from build123d import *

# Parameters (mm, degrees)
SKETCH1_W           = 28
SKETCH1_H           = 28
BOSS_EXTRUDE1_DEPTH = 25
SKETCH2_W           = 28
SKETCH2_H           = 22
CUT_EXTRUDE1_DEPTH  = 22
SKETCH3_W           = 6.8
SKETCH3_H           = 22
CUT_EXTRUDE2_DEPTH  = 46.299006612
SKETCH4_R           = 2.4
CUT_EXTRUDE3_DEPTH  = 44.508619836
SKETCH5_W           = 28
SKETCH5_H           = 6
CUT_EXTRUDE4_DEPTH  = 4
SKETCH6_W           = 2
SKETCH6_H           = 21
CUT_EXTRUDE5_DEPTH  = 45.821869662
SKETCH7_W           = 28
SKETCH7_H           = 26
BOSS_EXTRUDE2_DEPTH = 12
SKETCH9_W           = 6.8
SKETCH9_H           = 22
CUT_EXTRUDE6_DEPTH  = 12
SKETCH10_W          = 28
SKETCH10_H          = 22
CUT_EXTRUDE7_DEPTH  = 12


with BuildPart() as part:
    # Sketch1 → Boss-Extrude1 (new body)
    with BuildSketch(Plane(origin=(0, 0, 0), x_dir=(1, 0, 0), z_dir=(0, 1, 0))):
        with Locations((14, -14)):
            Rectangle(SKETCH1_W, SKETCH1_H)
    extrude(amount=BOSS_EXTRUDE1_DEPTH)

    # Sketch2 → Cut-Extrude1 (cut)
    with BuildSketch(Plane(origin=(0, 25, 0), x_dir=(1, 0, 0), z_dir=(0, 1, 0))):
        with Locations((14, -11)):
            Rectangle(SKETCH2_W, SKETCH2_H)
    extrude(amount=-CUT_EXTRUDE1_DEPTH, mode=Mode.SUBTRACT)

    # Sketch3 → Cut-Extrude2 (cut, through all)
    with BuildSketch(Plane(origin=(0, 3, 0), x_dir=(1, 0, 0), z_dir=(0, 1, 0))):
        with Locations((14, -11)):
            Rectangle(SKETCH3_W, SKETCH3_H)
    extrude(amount=-CUT_EXTRUDE2_DEPTH, mode=Mode.SUBTRACT)

    # Sketch4 → Cut-Extrude3 (cut, through all)
    with BuildSketch(Plane(origin=(0, 0, 22), x_dir=(-1, 0, 0), z_dir=(0, 0, -1))):
        with Locations((-14, 10)):
            Circle(SKETCH4_R)
    extrude(amount=-CUT_EXTRUDE3_DEPTH, mode=Mode.SUBTRACT)

    # Sketch5 → Cut-Extrude4 (cut)
    with BuildSketch(Plane(origin=(0, 25, 0), x_dir=(1, 0, 0), z_dir=(0, 1, 0))):
        with Locations((14, -25)):
            Rectangle(SKETCH5_W, SKETCH5_H)
    extrude(amount=-CUT_EXTRUDE4_DEPTH, mode=Mode.SUBTRACT)

    # Sketch6 → Cut-Extrude5 (cut, through all)
    with BuildSketch(Plane(origin=(28, 0, 0), x_dir=(0, 0, -1), z_dir=(1, 0, 0))):
        with Locations((-27, 10.5)):
            Rectangle(SKETCH6_W, SKETCH6_H)
    extrude(amount=-CUT_EXTRUDE5_DEPTH, mode=Mode.SUBTRACT)

    # Sketch7 → Boss-Extrude2 (add)
    with BuildSketch(Plane.XZ):
        with Locations((14, 13)):
            Rectangle(SKETCH7_W, SKETCH7_H)
    extrude(amount=BOSS_EXTRUDE2_DEPTH)

    # Sketch9 → Cut-Extrude6 (cut)
    with BuildSketch(Plane(origin=(0, 0, 0), x_dir=(1, 0, 0), z_dir=(0, 1, 0))):
        with Locations((14, -11)):
            Rectangle(SKETCH9_W, SKETCH9_H)
    extrude(amount=-CUT_EXTRUDE6_DEPTH, mode=Mode.SUBTRACT)

    # Sketch10 → Cut-Extrude7 (cut)
    with BuildSketch(Plane(origin=(0, 3, 0), x_dir=(1, 0, 0), z_dir=(0, 1, 0))):
        with Locations((14, -11)):
            Rectangle(SKETCH10_W, SKETCH10_H)
    extrude(amount=-CUT_EXTRUDE7_DEPTH, mode=Mode.SUBTRACT)


solid = part.part
Could you check a few things on this model? Use its own coordinates, in mm. A direction names the side the tool comes from. Round coordinates to 2 decimals unless told otherwise and drop trailing zeros. Order: outer loops, then holes, each group sorted by start corner. A loop starts at its lowest first (then second) coordinate and runs counter-clockwise, first axis right, second up.
Q1. Imagine slicing it at D-D, the plane y = 2. List the corners of the cut face in (x, z) for me.
Geometry says:
outline: (0, 22) - (28, 22) - (28, 26) - (0, 26) - close
Q2. Thinking about a two-plate mould opening in Y: for faces 1 (the face through (16.398, 10.106, 23.972)), 2 (the face through (14, 5, 22)), 3 (the face through (14, 21, 24)), which applies, released by +Y, released by -Y, zero draft, split by the parting line, or undercut?
Geometry says:
face 1: undercut
face 2: zero draft
face 3: released by +Y
Q3. Imagine slicing it at C-C, the plane x = 23.75. List the corners of the cut face in (y, z) for me.
Geometry says:
outline: (-12, 0) - (-9, 0) - (-9, 22) - (21, 22) - (21, 26) - (-12, 26) - close
Q4. I'm going to push flat-ended pins straight in: P1, Ø8, axis at x = 10, y = 11, coming from the -Z side; P2, Ø8.5, axis at x = 3, z = 6.5, coming from the +Y side; P3, Ø12, axis at y = 1, z = 7, coming from the +X side; P4, Ø7.5, axis at x = 14, y = 10, coming from the +Z side. Where does each tip first touch, or does it pass through?
Geometry says:
P1: stops at z = 22
P2: stops at y = -9
P3: passes through
P4: stops at z = 26
Q5. Which directions (+Z, -Z, +X, -X, +Y, -Y) give clear straight access to the entire face, cutting with the end or side of a thin tool? Please do faces 4 (the face through (8, -12, 13)), 5 (the face through (10.6, -10, 11)), 6 (the face through (23, -9, 11)).
Geometry says:
face 4: +Z, -Z, +X, -X, -Y
face 5: -Z, +Y, -Y
face 6: -Z, +X, -X, +Y
Q6. Imagine slicing it at A-A, the plane y = 10. List the corners of the cut face in (x, z) for me.
Geometry says:
outline: (0, 22) - (11.6, 22) - (11.6, 26) - (0, 26) - close; (16.4, 22) - (28, 22) - (28, 26) - (16.4, 26) - close
Q7. Imagine slicing it at B-B, the plane x = 14. List the corners of the cut face in (y, z) for me, then the cut area to 3 significant figures.
Geometry says:
outline: (-12, 22) - (7.6, 22) - (7.6, 26) - (-12, 26) - close; (12.4, 22) - (21, 22) - (21, 26) - (12.4, 26) - close
area: 113 mm2
Q8. Please list where these lines run through material, in increasing order: probe 1 along Y at (x, z) = (14, 24.35); probe 2 along X at (y, z) = (-10, 14.25); probe 3 along Y at (x, z) = (2.25, 6).
Geometry says:
probe 1: y = -12 to 7.6, 12.4 to 21
probe 2: x = 0 to 10.6, 17.4 to 28
probe 3: y = -12 to -9
